For this review, take the finished solid that the model builds, in its own axes (mm). Face numbers are marked on the shaded views. Coordinates: 2 decimals unless noted, no trailing zeros. Loops run counter-clockwise (first coordinate to the right, second up) from the corner with the lowest first, then second, coordinate; pieces in that order, holes last. Notation, with made-up numbers: M 20.5,-12 L 25.5,-12 A31 ccw 25.5,14 Z; hole C 77,-26.5 d8. An arc over 180 degrees is marked long. Put each result on its own line as item: value.
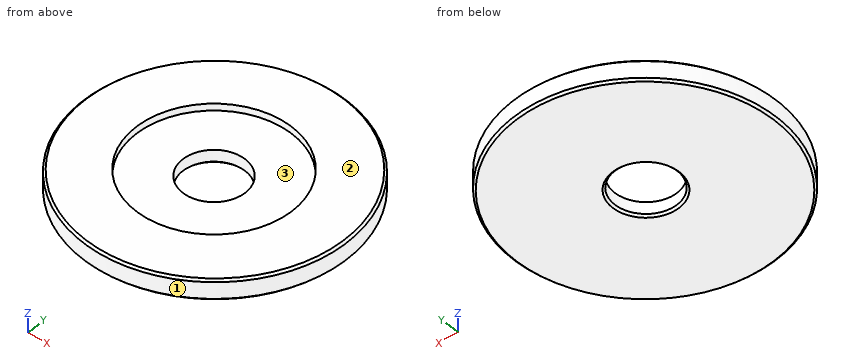
```python
from build123d import *

# Parameters (mm, degrees)
SKETCH043_R     = 19
PAD014_DEPTH    = 3
SKETCH044_R     = 4.5
POCKET030_DEPTH = 3.001
CHAMFER014_SIZE = 0.3
CHAMFER015_SIZE = 0.3
SKETCH057_R     = 11.25
POCKET037_DEPTH = 1


with BuildPart() as part:
    # Sketch043 → Pad014 (new body)
    with BuildSketch(Plane.XY):
        with Locations((0.140173, 0)):
            Circle(SKETCH043_R)
    extrude(amount=PAD014_DEPTH)

    # Sketch044 (on Face2 of Pad014) → Pocket030 (cut, through all)
    with BuildSketch(Plane(origin=(0, 0, 0), x_dir=(1, 0, 0), z_dir=(0, 0, -1))):
        Circle(SKETCH044_R)
    extrude(amount=-POCKET030_DEPTH, mode=Mode.SUBTRACT)

    # Chamfer014
    chamfer014_edges = [part.edges().sort_by_distance(p)[0] for p in [
        (-4.5, 0, 0),
        (-4.5, 0, 3),
    ]]
    chamfer(chamfer014_edges, length=CHAMFER014_SIZE)

    # Chamfer015
    chamfer015_edges = [part.edges().sort_by_distance(p)[0] for p in [
        (-18.859827, 0, 0),
        (-18.859827, 0, 3),
    ]]
    chamfer(chamfer015_edges, length=CHAMFER015_SIZE)

    # Sketch057 (on Face8 of Chamfer015) → Pocket037 (cut)
    with BuildSketch(Plane.XY.offset(3)):
        Circle(SKETCH057_R)
    extrude(amount=-POCKET037_DEPTH, mode=Mode.SUBTRACT)


solid = part.part
```
(1) For pin 1 (1.5 mm diameter, centred on y = 6.5, z = 2.5, fed in from +X); pin 2 (11 mm diameter, centred on x = 1.5, y = -4.5, fed in from +Z); pin 3 (1.5 mm diameter, centred on x = -10, y = -14, fed in from -Z); pin 4 (1 mm diameter, centred on y = -9.5, z = 0.5, fed in from +X), all flat-tipped, find the tip position at first contact; note any pin that passes through.
Determined:
pin 1: stops at x = 18.25
pin 2: stops at z = 2
pin 3: stops at z = 0
pin 4: stops at x = 16.87
(2) Add section A-A (y = 0). Write out the cut boundary in (x, z), plus the area to 3 significant figures.
Determined:
outline: M -18.86,0.3 L -18.56,0 L -4.8,0 L -4.5,0.3 L -4.5,2 L -11.25,2 L -11.25,3 L -18.56,3 L -18.86,2.7 Z; M 4.5,0.3 L 4.8,0 L 18.84,0 L 19.14,0.3 L 19.14,2.7 L 18.84,3 L 11.25,3 L 11.25,2 L 4.5,2 Z
area: 73.2 mm^2
(3) Wall thickness on line 1 along Y through (x, z) = (0, 0.8); line 2 along Z through (x, y) = (-4, 4); line 3 along Y through (x, z) = (0, 2.3): over which ranges is each line inside the solid? List them lowest first. Write a range as [from, to].
Determined:
line 1: y = [-19, -4.5], [4.5, 19]
line 2: z = [0, 2]
line 3: y = [-19, -11.25], [11.25, 19]
(4) Add section B-B (z = 1.4). Write out the cut boundary in (x, y), plus the area to 3 significant figures.
Determined:
outline: C 0.14,0 d38; hole C 0,0 d9
area: 1,070 mm^2
(5) Draft analysis for pull direction X (two halves, no side actions). For the marked faces 1, 2 and 3, state which applies: +X half, -X half, draft (parallel to the pull), parting line (faces both ways), or undercut.
Determined:
face 1: parting line
face 2: draft
face 3: undercut
